Verification items for the finished model (mm, model axes). Round coordinates to 2 decimals unless told otherwise and drop trailing zeros. Order: outer loops, then holes, each group sorted by start corner. A loop starts at its lowest first (then second) coordinate and runs counter-clockwise, first axis right, second up. Notation, with made-up numbers: (48, 11.5) -> (69, 11.5) arc R21 cw to (69, 45.5) -> close; hole circle Ø8 at (-36, 74.5). An arc over 180 degrees is marked (long way). Write item = value, one per line. Start each with the question number.
from build123d import *

# Parameters (mm, degrees)
BOSS_EXTRUDE1_DEPTH = 3.175
BOSS_EXTRUDE2_DEPTH = 3.175
SKETCH3_R           = 1.8288
CUT_EXTRUDE1_DEPTH  = 4.175
SKETCH5_R           = 1.27
CUT_EXTRUDE2_DEPTH  = 4.175


with BuildPart() as part:
    # Sketch1 → Boss-Extrude1 (new body)
    with BuildSketch(Plane(origin=(0, 0, 0), x_dir=(0, 0, -1), z_dir=(1, 0, 0))):
        with BuildLine():
            Line((0, 177.8), (0, 0))
            Line((0, 0), (177.8, 0))
            ThreePointArc((177.8, 0), (125.723585695, 125.723585695), (0, 177.8))
        make_face()
    extrude(amount=BOSS_EXTRUDE1_DEPTH)

    # Sketch2 → Boss-Extrude2 (add)
    with BuildSketch(Plane(origin=(3.175, 0, 0), x_dir=(0, 0, -1), z_dir=(1, 0, 0))):
        with BuildLine():
            Line((0, 0), (0, 12.7))
            ThreePointArc((0, 12.7), (-8.980256121, -8.980256121), (12.7, 0))
            Line((12.7, 0), (0, 0))
        make_face()
    extrude(amount=-BOSS_EXTRUDE2_DEPTH)

    # Sketch3 → Cut-Extrude1 (cut, through all)
    with BuildSketch(Plane(origin=(3.175, 0, 0), x_dir=(0, 0, -1), z_dir=(1, 0, 0))):
        with Locations((0, 9.779)):
            Circle(SKETCH3_R)
        with Locations((6.914797213, 6.914797213)):
            Circle(SKETCH3_R)
        with Locations((9.779, 0)):
            Circle(SKETCH3_R)
        with Locations((6.914797213, -6.914797213)):
            Circle(SKETCH3_R)
        with Locations((0, -9.779)):
            Circle(SKETCH3_R)
        with Locations((-6.914797213, -6.914797213)):
            Circle(SKETCH3_R)
        with Locations((-9.779, 0)):
            Circle(SKETCH3_R)
        with Locations((-6.914797213, 6.914797213)):
            Circle(SKETCH3_R)
    extrude(amount=-CUT_EXTRUDE1_DEPTH, mode=Mode.SUBTRACT)

    # Sketch5 → Cut-Extrude2 (cut, through all)
    with BuildSketch(Plane(origin=(3.175, 0, 0), x_dir=(0, 0, -1), z_dir=(1, 0, 0))):
        with Locations((163.159047333, 5.697639482)):
            Circle(SKETCH5_R)
    extrude(amount=-CUT_EXTRUDE2_DEPTH, mode=Mode.SUBTRACT)


solid = part.part
(1) Depth check by flat-ended pin: pin 1 (2 mm diameter, centred on y = 5.7, z = -163.16, fed in from -X); pin 2 (1.5 mm diameter, centred on x = 1.5, z = -50.5, fed in from -Y). Enter the tip coordinate at first touch or a pass-through.
(2) Cross-section at A-A (x = 2.5). Give the number of separate pieces and of enclosed holes in the cut face, and give its area (3 significant figures).
(3) Cross-section at B-B (y = 88). Enter the section's corners in (x, z) (3 decimals).
(4) Cross-section at C-C (z = -116.5). Enter the section's corners in (x, y) (3 decimals), and give its area (3 significant figures).
(5) Scan lines: line 1 along Z through (x, y) = (0.6, 6); line 2 along Y through (x, z) = (1.9, -7); line 3 along Z through (x, y) = (2, -0.5). Record each from-to range of solid material in increasing order. Write a range as from..to.
Outcome:
q1.pin_1 = through
q1.pin_2 = 0
q2.separate_pieces = 1
q2.enclosed_holes = 9
q2.area = 25,100 mm^2
q3.outline = (0, -154.495) -> (3.175, -154.495) -> (3.175, 0) -> (0, 0) -> close
q4.outline = (0, 0) -> (3.175, 0) -> (3.175, 134.315) -> (0, 134.315) -> close
q4.area = 426 mm^2
q5.line_1 = -177.7..-164.39, -161.93..-8.5, -5.33..5.33, 8.5..11.19
q5.line_2 = -10.6..-8.74, -5.09..5.09, 8.74..177.66
q5.line_3 = -12.69..-11.54, -8.02..8.02, 11.54..12.69
